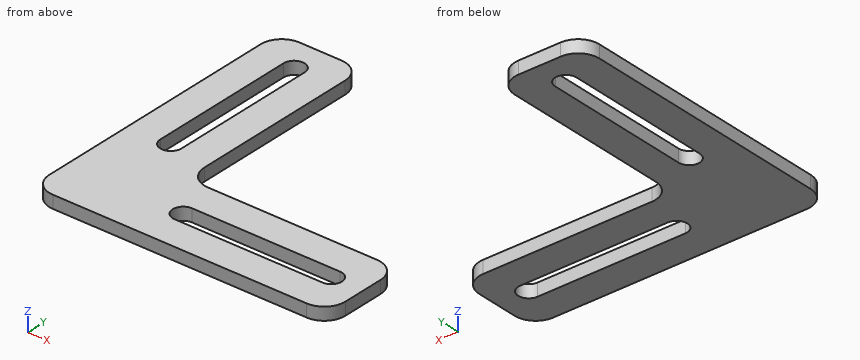
from build123d import *

# Parameters (mm, degrees)
BOSS_EXTRUDE1_DEPTH = 3
FILLET1_R           = 5


with BuildPart() as part:
    # Sketch1 → Boss-Extrude1 (new body)
    with BuildSketch(Plane.XY):
        Polygon((0, 70), (0, 0), (70, 0), (70, 20), (20, 20), (20, 70), align=None)
        with BuildLine():
            Line((12.5, 62.5), (12.5, 27.5))
            ThreePointArc((12.5, 27.5), (10, 25), (7.5, 27.5))
            Line((7.5, 27.5), (7.5, 62.5))
            ThreePointArc((7.5, 62.5), (10, 65), (12.5, 62.5))
        make_face(mode=Mode.SUBTRACT)
        with BuildLine():
            Line((62.5, 7.5), (27.5, 7.5))
            ThreePointArc((27.5, 7.5), (25, 10), (27.5, 12.5))
            Line((27.5, 12.5), (62.5, 12.5))
            ThreePointArc((62.5, 12.5), (65, 10), (62.5, 7.5))
        make_face(mode=Mode.SUBTRACT)
    extrude(amount=BOSS_EXTRUDE1_DEPTH)

    # Fillet1
    fillet1_edges = [part.edges().sort_by_distance(p)[0] for p in [
        (20, 70, 1.5),
        (20, 20, 1.5),
        (70, 20, 1.5),
        (70, 0, 1.5),
        (0, 0, 1.5),
        (0, 70, 1.5),
    ]]
    fillet(fillet1_edges, radius=FILLET1_R)


solid = part.part
Model file for the job. Use its own axes, mm. Give positions to 0.01 mm unless a question says otherwise; leave off trailing zeros. Order: outer loops, then holes, each group sorted by start corner. A loop starts at its lowest first (then second) coordinate and runs counter-clockwise, first axis right, second up. Notation, with made-up numbers: (0, -30.5) - (48, -30.5) arc R7 ccw to (48, -18.5) - close; hole circle Ø3 at (-4, -34). An arc over 180 degrees is marked (long way). Return JSON: item names as keys, results as strings.
1) Flat gauge pins, fed straight in: P1, Ø0.9, axis at y = 38.5, z = 1.5, coming from the +X side; P2, Ø1.5, axis at x = 53.5, z = 1.5, coming from the +Y side. Where does each tip first touch, or does it go through?
Geometry says:
{"P1": "x = 20", "P2": "y = 20"}
2) Cut at C-C, the plane z = 0.6. Give the cut face in (x, y), plus the area to 3 significant figures.
Geometry says:
{"outline": "(0, 5) arc R5 ccw to (5, 0) - (65, 0) arc R5 ccw to (70, 5) - (70, 15) arc R5 ccw to (65, 20) - (25, 20) arc R5 cw to (20, 25) - (20, 65) arc R5 ccw to (15, 70) - (5, 70) arc R5 ccw to (0, 65) - close; hole (7.5, 27.5) arc R2.5 ccw to (12.5, 27.5) - (12.5, 62.5) arc R2.5 ccw to (7.5, 62.5) - close; hole (27.5, 7.5) - (62.5, 7.5) arc R2.5 ccw to (62.5, 12.5) - (27.5, 12.5) arc R2.5 ccw to start", "area": "1,990 mm²"}
3) Cut at A-A, the plane y = 46. Give the cut face in (x, z), plus the area to 3 significant figures.
Geometry says:
{"outline": "(0, 0) - (7.5, 0) - (7.5, 3) - (0, 3) - close; (12.5, 0) - (20, 0) - (20, 3) - (12.5, 3) - close", "area": "45.0 mm²"}
4) Probe line 1 (X direction, y = 38, z = 1.5); line 2 (Y direction, x = 12, z = 1.5). List the from-to ranges inside material, lowest first. Write a range as from..to.
Geometry says:
{"line 1": "0..7.5, 12.5..20", "line 2": "0..26, 64..70"}
